Input: part model. Units: mm. Frame: model coordinates. A direction names the side the tool comes from. Coordinates: 2 decimals unless noted, no trailing zeros. Write each loop counter-clockwise with the first axis right and the second up, starting at its lowest first coordinate (ties: lowest second). Pieces come first, ordered by that corner, then holes. Notation, with made-up numbers: (-0.5, 43.5) - (7.5, 43.5) arc R14 ccw to (7.5, 49.5) - close; hole circle Ø9 at (73.25, 23). An arc over 180 degrees is marked (long way). Put each result on its own line as item: value. Start each with the question number.
1. Access query for faces 4 (the flat face through (22, 54, 10)), 5 (the flat face through (-30, 56, 8)), 6 (the cylindrical face through (29.54, 8.03, 26.53)), 7 (the flat face through (0, 43, 1.9)), 8 (the flat face through (-8.77, 55.22, -28.79)). Directions: +Z, -Z, +X, -X, +Y, -Y. A direction counts if a zero-diameter tool reaches every point of the face in a straight line with its end or side. Return the directions, or none.
2. Cut plane A-A, the plane z = 30. Return loops of the section in (x, y).
3. Cut plane C-C, the plane y = 26.5. Return loops of the section in (x, z).
4. Cut plane B-B, the plane x = 30. Return loops of the section in (y, z).
5. Line query: line 1 (X direction, y = 33, z = -16.5); line 2 (X direction, y = 3, z = 30). Output: solid intervals per line, ascending.
6. Pin query (flat end, axial travel): pin 1 (2 mm diameter, centred on x = 28.5, z = 31.5, fed in from +Y); pin 2 (3 mm diameter, centred on y = 59.5, z = -26.5, fed in from -X); pin 3 (1.5 mm diameter, centred on x = 3.5, z = -38.5, fed in from +Y); pin 4 (4.5 mm diameter, centred on x = 0.5, y = 41.5, fed in from +Z). Return the tip coordinate at first contact, or that it passes through.
7. Pull-direction query (X, two-part tool) for faces 1 (the flat face through (1, 5, -50)), 2 (the flat face through (50, 37, -10)), 3 (the flat face through (41.23, 55.22, -28.79)); classes: released by +X, released by -X, zero draft, split by the parting line, or undercut.
Autodesk Fusion 360 part; units mm, degrees
sketch "Sketch1" plane through (0, 0, 0) normal (0, 1, 0) x (1, 0, 0)
  line L0 (30, 30) -> (-30, 30)
  line L1 (-30, 30) -> (-30, -30)
  line L2 (-30, -30) -> (30, -30)
  line L3 (30, -30) -> (30, 30)
  line L4 (30, 30) -> (-30, -30) construction
  line L5 (-30, 30) -> (30, -30) construction
  circle A0 centre (-30, 30) radius 2.5
  circle A1 centre (30, 30) radius 2.5
  circle A2 centre (-30, -30) radius 2.5
  circle A3 centre (30, -30) radius 2.5
  line L6 (50, 50) -> (-50, 50)
  line L7 (-50, 50) -> (-50, -50)
  line L8 (-50, -50) -> (50, -50)
  line L9 (50, -50) -> (50, 50)
  line L10 (50, 50) -> (-50, -50) construction
  line L11 (-50, 50) -> (50, -50) construction
  line L12 (50, 10) -> (-50, 10)
  line L13 (-50, 10) -> (-50, -10)
  line L14 (-50, -10) -> (50, -10)
  line L15 (50, -10) -> (50, 10)
  line L16 (50, 10) -> (-50, -10) construction
  line L17 (-50, 10) -> (50, -10) construction
  circle A4 centre (-30, -30) radius 3.5
  circle A5 centre (30, -30) radius 3.5
  dimension "d1" = 60
  dimension "d2" = 60
  dimension "d3" = 5
  dimension "d6" = 60
  dimension "d7" = -60
  dimension "d8" = 100
  dimension "d9" = 100
  dimension "d10" = 100
  dimension "d11" = 20
  dimension "d49" = 7
  dimension "d50" = 7
extrude "Extrude1" add sketch "Sketch1" along normal blind 10 contours L0 L1 L3 A0 A1 L6 L7 L9 L12 | L0 L1 L3 A0 A1 L12 | L1 L3 L12 L14 | L1 L7 L12 L13 L14 | L3 L9 L12 L14 L15 | L1 L2 L3 L14 A4 A5 | L1 L2 L3 L7 L8 L9 L14 A4 A5 | L1 L2 A2 A4 | L1 L2 A2 A4 | L2 L3 A3 A5 | L2 L3 A3 A5
extrude "Extrude2" add sketch "Sketch1" along normal blind 90 from surface at 10 contours L1 L3 L12 L14 | L1 L7 L12 L13 L14 | L3 L9 L12 L14 L15
sketch "Sketch2" plane through (0, 0, -10) normal (0, 0, -1) x (-1, 0, 0)
  line L0 (-50, 10) -> (50, 10)
  line L1 (50, 10) -> (50, 100)
  line L2 (50, 100) -> (-50, 100)
  line L3 (-50, 100) -> (-50, 10)
  line L4 (-50, 100) -> (-40, 100)
  line L5 (-40, 100) -> (-40, 10)
  line L6 (-40, 10) -> (-50, 10)
  line L7 (-50, 10) -> (-50, 100)
  line L8 (50, 100) -> (40, 100)
  line L9 (40, 100) -> (40, 10)
  line L10 (40, 10) -> (50, 10)
  line L11 (50, 10) -> (50, 100)
  line L12 (0, 100) -> (0, 10)
  line L13 (10, 100) -> (-10, 100)
  line L14 (-10, 100) -> (-10, 10)
  line L15 (-10, 10) -> (10, 10)
  line L16 (10, 10) -> (10, 100)
  dimension "d17" = 10
  dimension "d19" = 10
  dimension "d22" = 20
  dimension "d23" = 20
extrude "Extrude3" add sketch "Sketch2" along normal up to surface (40 mm away) contours L0 L2 L3 L4 L5 L6 L7 | L0 L2 L12 L13 L14 L15 | L0 L2 L12 L13 L15 L16 | L0 L1 L2 L8 L9 L10 L11
chamfer "Chamfer1" distance 40 distance2 90 3 edges at (45, 100, -50) (0, 100, -50) (-45, 100, -50) measured on face at (-3.3333, 100, 3.3333) measured on face at (-3.3333, 100, 3.3333) measured on face at (-3.3333, 100, 3.3333)
chamfer "Chamfer2" distance 2.5 distance2 2 6 edges at (50, 55, -30) (40, 55, -30) (10, 55, -30) (-10, 55, -30) (-40, 55, -30) (-50, 55, -30) measured on face at (43.3333, 40, -36.6667) measured on face at (43.3333, 40, -36.6667) measured on face at (3.3333, 40, -36.6667) measured on face at (3.3333, 40, -36.6667) measured on face at (-43.3333, 70, -23.3333) measured on face at (-43.3333, 70, -23.3333)
chamfer "Chamfer3" distance 2.5 distance2 2 2 edges at (50, 100, 1.0943) (-50, 100, 1.0943) measured on face at (-2.5, 100, 3.3333) measured on face at (-50, 38.3585, -15.9371)
sketch "Sketch3" plane through (0, 0, 10) normal (0, 0, 1) x (1, 0, 0)
  line L0 (-48, 100) -> (-50, 97.5)
  line L1 (-50, 97.5) -> (-50, 10)
  line L2 (-50, 10) -> (50, 10)
  line L3 (50, 10) -> (50, 98)
  line L4 (50, 98) -> (47.5, 100)
  line L5 (47.5, 100) -> (-48, 100)
  line L6 (-0.25, 100) -> (0, 10)
  line L7 (-50, 10) -> (50, 10)
  line L8 (50, 10) -> (50, 100)
  line L9 (50, 100) -> (-50, 100)
  line L10 (-50, 100) -> (-50, 10)
  line L11 (50, 55) -> (-50, 55) construction
  circle A0 centre (-0.0903, 42.5) radius 2.8
  circle A1 centre (-0.0903, 67.5) radius 2.8
  line L12 (-50, 12.5) -> (-10.0903, 12.5)
  line L13 (-10.0903, 12.5) -> (-10.0903, 97.5)
  line L14 (-10.0903, 97.5) -> (-50, 97.5)
  line L15 (-50, 97.5) -> (-50, 12.5)
  dimension "d43" = 90
  dimension "d44" = 100
  dimension "d45" = 5.6
  dimension "d46" = 12.5
  dimension "d54" = 85
  dimension "d55" = 10
extrude "Extrude4" cut sketch "Sketch3" against normal blind 8.1 contours L6 A1 | L6 A1 | L6 A0 | L6 A0
extrude "Extrude5" cut sketch "Sketch1" against normal blind 4 from surface at 10 contours L1 L2 A2 A4 | L1 L2 A2 A4 | L2 L3 A3 A5 | L2 L3 A3 A5
extrude "Extrude6" cut sketch "Sketch3" against normal blind 2 contours L1 L10 L12 L13 L14 L15
chamfer "Chamfer4" distance 2 angle 45 1 edges at (-30.0451, 97.5, 10)
equation "d46 = ( 25 / 2 ) * 1 mm"
Report:
1. face 4: +Z, +X, -X, +Y
1. face 5: +Z, -X
1. face 6: +Y
1. face 7: +Z
1. face 8: -Z, +Y
2. outline: (-50, 0) - (-32.5, 0) - (-32.5, 6) - (-33.5, 6) - (-33.5, 10) - (-50, 10) - close; (-27.5, 0) - (27.5, 0) - (27.5, 6) - (26.5, 6) - (26.5, 10) - (-26.5, 10) - (-26.5, 6) - (-27.5, 6) - close; (32.5, 0) - (50, 0) - (50, 10) - (33.5, 10) - (33.5, 6) - (32.5, 6) - close
3. outline: (-50, -40.48) - (-47.5, -42.67) - (-42.5, -42.67) - (-40, -40.48) - (-40, -10) - (-10, -10) - (-10, -40.48) - (-7.5, -42.67) - (7.5, -42.67) - (10, -40.48) - (10, -10) - (40, -10) - (40, -40.48) - (42.5, -42.67) - (47.5, -42.67) - (50, -40.48) - (50, 10) - (-10.09, 10) - (-10.09, 8) - (-50, 8) - close
4. outline: (0, -50) - (10, -50) - (10, -32.5) - (0, -32.5) - close; (0, -27.5) - (10, -27.5) - (10, -10) - (100, -10) - (100, 10) - (10, 10) - (10, 26.5) - (6, 26.5) - (6, 27.5) - (0, 27.5) - close; (0, 32.5) - (6, 32.5) - (6, 33.5) - (10, 33.5) - (10, 50) - (0, 50) - close
5. line 1: x = -50 to -40, -10 to 10, 40 to 50
5. line 2: x = -50 to -32.5, -27.5 to 27.5, 32.5 to 50
6. pin 1: stops at y = 6
6. pin 2: stops at x = -50
6. pin 3: stops at y = 37.56
6. pin 4: stops at z = 10
7. face 1: zero draft
7. face 2: released by +X
7. face 3: undercut
